```python
from build123d import *

# Parameters (mm, degrees)
F0_R        = 13.5872580749
F1_DEPTH    = 16.764
F2_W        = 11.076066643
F2_H        = 72.8688556701
F3_DEPTH    = 63.754
F4_SIZE2    = 40.64
F4_SIZE     = 30.48
F5_W        = 49.8422943056
F5_H        = 10.4931145906
F6_DEPTH    = 64.008
F7_T4_DEPTH = 271.9527686037


# Not quite as in the source:
# - a fillet or chamfer that OpenCascade refuses, or shapes differently, is made with other operations: its cross-section is extruded or revolved along the edge and cut away or added


with BuildPart() as f1:
    # F0 (on Front) → F1 (new body)
    with BuildSketch(Plane.XZ):
        Polygon((-29.1315091585, 37.5352683077), (-60.8815091585, 37.5352683077), (-60.8815091585, -51.3647316923), (53.4184908415, -51.3647316923), (53.4184908415, -11.1139282757), align=None)
        with Locations((28.8560632616, -24.9211471528)):
            Circle(F0_R, mode=Mode.SUBTRACT)
    extrude(amount=F1_DEPTH)

    # F2 (on Front) → F3 (join)
    with BuildSketch(Plane.XZ):
        with Locations((-55.6718055159, -14.4280334935)):
            Rectangle(F2_W, F2_H)
    extrude(amount=F3_DEPTH)

    # F4
    f4_edges = [f1.edges().sort_by_distance(p)[0] for p in [
        (-55.671806, -63.754, 22.006394),
    ]]
    f4_side = f1.faces().sort_by_distance((-55.728042, -39.925416, 22.006394))[0]
    chamfer(f4_edges, length=F4_SIZE, length2=F4_SIZE2, reference=f4_side)

    # F5 (on Front) → F6 (join)
    with BuildSketch(Plane.XZ):
        with Locations((-24.9211471528, -45.3244261444)):
            Rectangle(F5_W, F5_H)
    extrude(amount=F6_DEPTH)

    # F7: chamfer of 48.26 x 50.8 on 1 edges, made by hand


with BuildPart() as f7_tool2:
    # F7_s3 → F7_t4 (new body)
    with BuildSketch(Plane.XY.offset(-181.3008104462)):
        Polygon((0, -15.748), (-50.8, -64.008), (0, -64.008), align=None)
    extrude(amount=F7_T4_DEPTH)

    split(bisect_by=Plane.XZ.offset(16.764), keep=Keep.TOP)

    split(bisect_by=Plane.YZ.offset(-49.8422943056), keep=Keep.TOP)


with BuildPart() as f1_1:
    add(f1.part)

    # F7_t1: cut F7_tool2
    add(f7_tool2.part, mode=Mode.SUBTRACT)


solid = f1_1.part
```
Source: CAD feature listing. Evaluate the final solid. Frame: model axes, mm. A direction names the side the tool comes from. Round coordinates to 2 decimals unless told otherwise and drop trailing zeros. Order: outer loops, then holes, each group sorted by start corner. A loop starts at its lowest first (then second) coordinate and runs counter-clockwise, first axis right, second up. Notation, with made-up numbers: (-18.75, 36.5) -> (0.25, 36.5) arc R16 cw to (0.25, 59.5) -> close; hole circle Ø1 at (12, -31.75). An arc over 180 degrees is marked (long way). One line per item, written item: value. Start each with the question number.
Q1. Draft query along X for faces 1 (the flat face through (-61.21, -31, -15)), 2 (the cylindrical face through (35.126, -8.265, -36.975)), 3 (the flat face through (-5, -8, -51.365)). Return one class per face: pulls with the +X half, pulls with the -X half, needs draft (parallel to the pull), parting line crosses it, or undercut.
Q2. Pin query (flat end, axial travel): pin 1 (14 mm diameter, centred on x = -17.5, y = -41, fed in from -Z); pin 2 (16.5 mm diameter, centred on x = 28.86, z = -24.92, fed in from -Y); pin 3 (4 mm diameter, centred on y = -50, z = -22, fed in from +X); pin 4 (14 mm diameter, centred on x = -27.5, y = -32.5, fed in from +Z). Return the tip coordinate at first contact, or that it passes through.
Q3. Section query D-D (y = -38). Return the cut outline in (x, z).
Q4. Access query for faces 4 (the flat face through (-31, -34, -50.571)), 5 (the flat face through (-50.134, -35, -23)), 6 (the flat face through (-31, -34, -40.078)), 7 (the flat face through (-60.882, -8, 30)). Directions: +Z, -Z, +X, -X, +Y, -Y. A direction counts if a zero-diameter tool reaches every point of the face in a straight line with its end or side. Return the directions, or none.
Q5. Section query A-A (z = -28). Return the cut outline in (x, y).
Q6. Section query C-C (x = -53.5). Return the cut outline in (y, z).
Q7. Material intervals for probe 1 along Y at (x, z) = (-36, 20.5); probe 2 along Z at (x, y) = (22, -8.5); probe 3 along X at (y, z) = (-49, -41.5), sorted ascending.
Q8. Section query B-B (y = -46.5). Return the cut outline in (x, z), plus the area to 3 significant figures.
Findings below:
1. face 1: pulls with the -X half
1. face 2: undercut
1. face 3: needs draft
2. pin 1: z = -50.57
2. pin 2: through
2. pin 3: x = -50.13
2. pin 4: z = -40.08
3. outline: (-61.21, -50.86) -> (-50.13, -50.86) -> (-50.13, 15.71) -> (-61.21, 15.71) -> close; (-49.84, -50.57) -> (-23.42, -50.57) -> (-23.42, -40.08) -> (-49.84, -40.08) -> close
4. face 4: -Z, +X, -Y
4. face 5: +Z, -Z, -Y
4. face 6: +Z, +X, -Y
4. face 7: +Z, -X, +Y, -Y
5. outline: (-61.21, -63.75) -> (-50.13, -63.75) -> (-50.13, -16.76) -> (15.62, -16.76) -> (15.62, 0) -> (-61.21, 0) -> close; (42.09, -16.76) -> (53.42, -16.76) -> (53.42, 0) -> (42.09, 0) -> close
6. outline: (-63.75, -50.86) -> (-16.76, -50.86) -> (-16.76, -51.36) -> (0, -51.36) -> (0, 37.54) -> (-16.76, 37.54) -> (-16.76, 22.01) -> (-33.27, 22.01) -> (-63.75, -18.63) -> close
7. probe 1: -16.76 to 0
7. probe 2: -51.36 to -36.65, -13.19 to 7.4
7. probe 3: -61.21 to -50.13, -49.84 to -35
8. outline: (-61.21, -50.86) -> (-50.13, -50.86) -> (-50.13, 4.37) -> (-61.21, 4.37) -> close; (-49.84, -50.57) -> (-32.37, -50.57) -> (-32.37, -40.08) -> (-49.84, -40.08) -> close
8. area: 795 mm²
